```python
from build123d import *

# Parameters (mm, degrees)
F0_W     = 100
F0_H     = 35
F1_DEPTH = 1.5
F2_W     = 100
F2_H     = 2
F3_DEPTH = 28


with BuildPart() as f1:
    # F0 (on Front) → F1 (new body)
    with BuildSketch(Plane.XZ):
        Rectangle(F0_W, F0_H)
    extrude(amount=F1_DEPTH)

    # F2 (on face) → F3 (join)
    with BuildSketch(Plane.XZ.offset(1.5)):
        with Locations((-1e-06, 13.460001)):
            Rectangle(F2_W, F2_H)
    extrude(amount=F3_DEPTH)


solid = f1.part
```
Check sheet for the modelled part. Datum: model origin and axes. Units: mm. A direction names the side the tool comes from. Give positions to 0.01 mm unless a question says otherwise; leave off trailing zeros. Write each loop counter-clockwise with the first axis right and the second up, starting at its lowest first coordinate (ties: lowest second). Pieces come first, ordered by that corner, then holes.
Item 1: Cross-section at A-A (x = 34.5). Enter the section's corners in (y, z), and give its area (4 significant figures).
Item 2: Scan lines: L1, parallel to Z at x = 27.5, y = -20.25; L2, parallel to Y at x = -11, z = 9. Record each from-to range of solid material in increasing order.
Item 3: Gauge pin test, flat ends, axial feed: pin 1 (8 mm diameter, centred on x = -21, z = -12.5, fed in from +Y); pin 2 (12 mm diameter, centred on x = -4, y = -9, fed in from +Z); pin 3 (10 mm diameter, centred on x = 6, z = -13, fed in from -Y); pin 4 (14 mm diameter, centred on x = -7, y = -19, fed in from -Z). Record the tip position at first contact, or that the pin passes through.
Item 4: Cross-section at C-C (y = -11). Enter the section's corners in (x, z), and give its area (3 significant figures).
Item 5: Cross-section at B-B (z = -4). Enter the section's corners in (x, y), and give its area (3 significant figures).
Item 6: Access from +Z, -Z, +X, -X, +Y, -Y to the whole of each face (thin tool, end or side, straight path). Record for faces 1 (the face through (-50, -15, 13)), 2 (the face through (-1, -15, 14.46)), 3 (the face through (-1, -15, 12.46)).
Report:
1. outline: (-29.5, 12.46) - (-1.5, 12.46) - (-1.5, -17.5) - (0, -17.5) - (0, 17.5) - (-1.5, 17.5) - (-1.5, 14.46) - (-29.5, 14.46) - close
1. area: 108.5 mm2
2. L1: z = 12.46 to 14.46
2. L2: y = -1.5 to 0
3. pin 1: stops at y = 0
3. pin 2: stops at z = 14.46
3. pin 3: stops at y = -1.5
3. pin 4: stops at z = 12.46
4. outline: (-50, 12.46) - (50, 12.46) - (50, 14.46) - (-50, 14.46) - close
4. area: 200 mm2
5. outline: (-50, -1.5) - (50, -1.5) - (50, 0) - (-50, 0) - close
5. area: 150 mm2
6. face 1: +Z, -Z, -X, +Y, -Y
6. face 2: +Z, +X, -X, -Y
6. face 3: -Z, +X, -X, -Y
